```python
from build123d import *

# Parameters (mm, degrees)
SKETCH1_W                       = 40
SKETCH1_H                       = 44
BOSS_EXTRUDE1_DEPTH             = 8
SKETCH2_W                       = 8.2
SKETCH2_H                       = 10
CUT_EXTRUDE1_DEPTH              = 1
SKETCH3_W                       = 8.2
SKETCH3_H                       = 8.2
CUT_EXTRUDE2_DEPTH              = 4
CHAMFER1_SIZE                   = 1
SKETCH4_R                       = 1.65
CUT_EXTRUDE3_DEPTH              = 56.398555938
SKETCH5_W                       = 17.6
SKETCH5_H                       = 3.725
BOSS_EXTRUDE2_DEPTH             = 8.5
BOSS_EXTRUDE2_DIRECTION_2_REACH = 57.749
FILLET1_R                       = 4
SKETCH6_R                       = 1.4
CUT_EXTRUDE4_DEPTH              = 10
CHAMFER2_SIZE                   = 2


with BuildPart() as part:
    # Sketch1 → Boss-Extrude1 (new body)
    with BuildSketch(Plane.XY):
        with Locations((20, 16)):
            Rectangle(SKETCH1_W, SKETCH1_H)
    extrude(amount=BOSS_EXTRUDE1_DEPTH)

    # Sketch2 → Cut-Extrude1 (cut)
    with BuildSketch(Plane.XY.offset(8)):
        with Locations((20, 31)):
            Rectangle(SKETCH2_W, SKETCH2_H)
        with Locations((6.1, 1)):
            Rectangle(SKETCH2_W, SKETCH2_H)
        with Locations((33.9, 1)):
            Rectangle(SKETCH2_W, SKETCH2_H)
    extrude(amount=-CUT_EXTRUDE1_DEPTH, mode=Mode.SUBTRACT)

    # Sketch3 → Cut-Extrude2 (cut)
    with BuildSketch(Plane.XY.offset(7)):
        with Locations((20, 31)):
            Rectangle(SKETCH3_W, SKETCH3_H)
        with Locations((6.1, 1)):
            Rectangle(SKETCH3_W, SKETCH3_H)
        with Locations((33.9, 1)):
            Rectangle(SKETCH3_W, SKETCH3_H)
    extrude(amount=-CUT_EXTRUDE2_DEPTH, mode=Mode.SUBTRACT)

    # Chamfer1
    chamfer1_edges = [part.edges().sort_by_distance(p)[0] for p in [
        (20, 26, 8),
        (20, 36, 8),
        (33.9, -4, 8),
        (33.9, 6, 8),
        (6.1, -4, 8),
        (6.1, 6, 8),
    ]]
    chamfer(chamfer1_edges, length=CHAMFER1_SIZE - 0.0001)  # a hair under: the kernel refuses the full size

    # Sketch4 → Cut-Extrude3 (cut, through all)
    with BuildSketch(Plane.XY.offset(3)):
        with Locations((20, 31)):
            Circle(SKETCH4_R)
        with Locations((6.1, 1)):
            Circle(SKETCH4_R)
        with Locations((33.9, 1)):
            Circle(SKETCH4_R)
    extrude(amount=-CUT_EXTRUDE3_DEPTH, mode=Mode.SUBTRACT)

    # Sketch5 → Boss-Extrude2 (add)
    with BuildSketch(Plane.XY.offset(8)):
        Polygon((20.704347826, 11.125), (19.295652174, 11.125), (18.695652174, 9.944955324), (16.695652174, 9.944955324), (16.095652174, 11.125), (15.195652174, 11.125), (13.786956522, 11.125), (13.186956522, 9.944955324), (11.186956522, 9.944955324), (10.586956522, 11.125), (9.686956522, 11.125), (8.27826087, 11.125), (7.67826087, 9.944955324), (5.67826087, 9.944955324), (5.07826087, 11.125), (4.17826087, 11.125), (0, 11.125), (0, 19), (40, 19), (40, 11.125), (35.82173913, 11.125), (34.92173913, 11.125), (34.32173913, 9.944955324), (32.32173913, 9.944955324), (31.72173913, 11.125), (30.313043478, 11.125), (29.413043478, 11.125), (28.813043478, 9.944955324), (26.813043478, 9.944955324), (26.213043478, 11.125), (24.804347826, 11.125), (23.904347826, 11.125), (23.304347826, 9.944955324), (21.304347826, 9.944955324), align=None)
        with Locations((20, 6.8625)):
            Rectangle(SKETCH5_W, SKETCH5_H)
        Polygon((0, 35), (14.9, 35), (14.9, 38), (10, 41), (5, 41), (0, 38), align=None)
        Polygon((25.1, 38), (30, 41), (35, 41), (40, 38), (40, 35), (25.1, 35), align=None)
    extrude(amount=BOSS_EXTRUDE2_DEPTH)

    # Boss-Extrude2 direction 2: up to this face of the body (flat: up to its plane)
    boss_extrude2_direction_2_end = Plane(part.part.faces().sort_by_distance((20, 16.073973219, 0))[0])
    # Sketch5 → Boss-Extrude2 direction 2 (add, up to the picked face)
    with BuildSketch(Plane.XY.offset(8), mode=Mode.PRIVATE) as boss_extrude2_direction_2_sk1:
        Polygon((20.704347826, 11.125), (19.295652174, 11.125), (18.695652174, 9.944955324), (16.695652174, 9.944955324), (16.095652174, 11.125), (15.195652174, 11.125), (13.786956522, 11.125), (13.186956522, 9.944955324), (11.186956522, 9.944955324), (10.586956522, 11.125), (9.686956522, 11.125), (8.27826087, 11.125), (7.67826087, 9.944955324), (5.67826087, 9.944955324), (5.07826087, 11.125), (4.17826087, 11.125), (0, 11.125), (0, 19), (40, 19), (40, 11.125), (35.82173913, 11.125), (34.92173913, 11.125), (34.32173913, 9.944955324), (32.32173913, 9.944955324), (31.72173913, 11.125), (30.313043478, 11.125), (29.413043478, 11.125), (28.813043478, 9.944955324), (26.813043478, 9.944955324), (26.213043478, 11.125), (24.804347826, 11.125), (23.904347826, 11.125), (23.304347826, 9.944955324), (21.304347826, 9.944955324), align=None)
    boss_extrude2_direction_2_tool1 = split(extrude(boss_extrude2_direction_2_sk1.sketch, amount=-BOSS_EXTRUDE2_DIRECTION_2_REACH, mode=Mode.PRIVATE), bisect_by=boss_extrude2_direction_2_end, keep=Keep.BOTH, mode=Mode.PRIVATE)
    # Sketch5 → Boss-Extrude2 direction 2 (add, up to the picked face)
    with BuildSketch(Plane.XY.offset(8), mode=Mode.PRIVATE) as boss_extrude2_direction_2_sk2:
        with Locations((20, 6.8625)):
            Rectangle(SKETCH5_W, SKETCH5_H)
    boss_extrude2_direction_2_tool2 = split(extrude(boss_extrude2_direction_2_sk2.sketch, amount=-BOSS_EXTRUDE2_DIRECTION_2_REACH, mode=Mode.PRIVATE), bisect_by=boss_extrude2_direction_2_end, keep=Keep.BOTH, mode=Mode.PRIVATE)
    # Sketch5 → Boss-Extrude2 direction 2 (add, up to the picked face)
    with BuildSketch(Plane.XY.offset(8), mode=Mode.PRIVATE) as boss_extrude2_direction_2_sk3:
        Polygon((0, 35), (14.9, 35), (14.9, 38), (10, 41), (5, 41), (0, 38), align=None)
    boss_extrude2_direction_2_tool3 = split(extrude(boss_extrude2_direction_2_sk3.sketch, amount=-BOSS_EXTRUDE2_DIRECTION_2_REACH, mode=Mode.PRIVATE), bisect_by=boss_extrude2_direction_2_end, keep=Keep.BOTH, mode=Mode.PRIVATE)
    # Sketch5 → Boss-Extrude2 direction 2 (add, up to the picked face)
    with BuildSketch(Plane.XY.offset(8), mode=Mode.PRIVATE) as boss_extrude2_direction_2_sk4:
        Polygon((25.1, 38), (30, 41), (35, 41), (40, 38), (40, 35), (25.1, 35), align=None)
    boss_extrude2_direction_2_tool4 = split(extrude(boss_extrude2_direction_2_sk4.sketch, amount=-BOSS_EXTRUDE2_DIRECTION_2_REACH, mode=Mode.PRIVATE), bisect_by=boss_extrude2_direction_2_end, keep=Keep.BOTH, mode=Mode.PRIVATE)
    add(boss_extrude2_direction_2_tool1.solids().sort_by(Axis((20, 14.815025, 8), (0, 0, -1)))[0])
    add(boss_extrude2_direction_2_tool2.solids().sort_by(Axis((20, 6.8625, 8), (0, 0, -1)))[0])
    add(boss_extrude2_direction_2_tool3.solids().sort_by(Axis((7.45835, 37.60161, 8), (0, 0, -1)))[0])
    add(boss_extrude2_direction_2_tool4.solids().sort_by(Axis((32.54165, 37.60161, 8), (0, 0, -1)))[0])

    # Fillet1
    fillet1_edges = [part.edges().sort_by_distance(p)[0] for p in [
        (20, 5, 8),
        (7.45, 35, 8),
        (32.55, 35, 8),
    ]]
    fillet(fillet1_edges, radius=FILLET1_R)

    # Sketch6 → Cut-Extrude4 (cut)
    with BuildSketch(Plane.XY.offset(16.5)):
        with Locations((7.5, 38)):
            Circle(SKETCH6_R)
        with Locations((7.5, 15)):
            Circle(SKETCH6_R)
        with Locations(Location((32.5, 38, 0), (0, 0, 180))):
            Circle(SKETCH6_R)
        with Locations(Location((32.5, 15, 0), (0, 0, 180))):
            Circle(SKETCH6_R)
    extrude(amount=-CUT_EXTRUDE4_DEPTH, mode=Mode.SUBTRACT)

    # Chamfer2
    chamfer2_edges = [part.edges().sort_by_distance(p)[0] for p in [
        (0, 11.125, 12.25),
        (0, 19, 12.25),
        (40, 19, 12.25),
        (40, 11.125, 12.25),
    ]]
    chamfer(chamfer2_edges, length=CHAMFER2_SIZE)


solid = part.part
```
The model under review builds one solid part; all positions refer to its coordinate system, in mm. A direction names the side the tool comes from. Give positions to 0.01 mm unless a question says otherwise; leave off trailing zeros. Write each loop counter-clockwise with the first axis right and the second up, starting at its lowest first coordinate (ties: lowest second). Pieces come first, ordered by that corner, then holes. Notation, with made-up numbers: M -15.5,8 L 31.5,8 A26 ccw 31.5,40 Z; hole C 58,2.5 d5. An arc over 180 degrees is marked long. Answer in a Markdown table with one row per item.
Item 1: For line 1 along Y through (x, z) = (7.5, 12.75); line 2 along Y through (x, z) = (8, 4.75); line 3 along Y through (x, z) = (32.5, 10.25), list the stretches that pass through material, from the lowest coordinate up.
Check sheet entries:
| item | result |
|---|---|
| line 1 | 9.94 to 13.6, 16.4 to 19, 35 to 36.6, 39.4 to 41 |
| line 2 | -6 to -3.1, 5.1 to 41 |
| line 3 | 9.94 to 13.6, 16.4 to 19, 34.6 to 36.6, 39.4 to 41 |
Item 2: For P1, Ø0.7, axis at x = 19, y = 26.5, coming from the +Z side; P2, Ø2, axis at x = 32.5, y = 15, coming from the +Z side; P3, Ø4.5, axis at x = 21.5, z = 5, coming from the +Y side, all flat-tipped, find the tip position at first contact; note any pin that passes through.
Check sheet entries:
| item | result |
|---|---|
| P1 | z = 7 |
| P2 | z = 6.5 |
| P3 | y = 38 |
Item 3: Add section B-B on y = 15. Give the boundary of the cut face in (x, z), plus the area to 3 significant figures.
Check sheet entries:
| item | result |
|---|---|
| outline | M 0,0 L 40,0 L 40,16.5 L 33.9,16.5 L 33.9,6.5 L 31.1,6.5 L 31.1,16.5 L 8.9,16.5 L 8.9,6.5 L 6.1,6.5 L 6.1,16.5 L 0,16.5 Z |
| area | 604 mm2 |
Item 4: Add section D-D on y = 28. Give the boundary of the cut face in (x, z).
Check sheet entries:
| item | result |
|---|---|
| outline | M 0,0 L 40,0 L 40,8 L 24.1,8 L 24.1,3 L 15.9,3 L 15.9,8 L 0,8 Z |
Item 5: Add section C-C on z = 10. State how many separate pieces and enclosed holes the cut face has, plus the area to 3 significant figures.
Check sheet entries:
| item | result |
|---|---|
| separate pieces | 4 |
| enclosed holes | 4 |
| area | 541 mm2 |
Item 6: Draft analysis for pull direction Y (two halves, no side actions). For faces 6 (the face through (6, 5.1, 5)), 7 (the face through (14.9, 36, 12)), 8 (the face through (7, 9.945, 12)), state which applies: +Y half, -Y half, draft (parallel to the pull), parting line (faces both ways), or undercut.
Check sheet entries:
| item | result |
|---|---|
| face 6 | undercut |
| face 7 | draft |
| face 8 | -Y half |
Item 7: Tool access review of faces 1 (the face through (25.1, 36, 12)), 2 (the face through (27.52, 39.48, 8.37)), 3 (the face through (36, 1, 3)), 4 (the face through (1, 18, 12)), 5 (the face through (31, 11.125, 12)): name each direction out of +Z, -Z, +X, -X, +Y, -Y from which nothing blocks a thin tool from reaching the whole face with its end or side.
Check sheet entries:
| item | result |
|---|---|
| face 1 | +Z, +Y |
| face 2 | +Z, -Z, +Y |
| face 3 | +Z |
| face 4 | +Z, -X |
| face 5 | +Z, -Y |
